Work out the finished part from the listing and answer in its coordinate system (mm). A direction names the side the tool comes from. Round coordinates to 2 decimals unless told otherwise and drop trailing zeros. Order: outer loops, then holes, each group sorted by start corner. A loop starts at its lowest first (then second) coordinate and runs counter-clockwise, first axis right, second up. Notation, with made-up numbers: (68.25, 59.25) - (116.25, 59.25) arc R21 ccw to (116.25, 84.25) - close; hole circle Ø5 at (-18.75, 18). An arc over 180 degrees is marked (long way). Put each result on its own line as item: value.
```python
from build123d import *

# Parameters (mm, degrees)
SKETCH1_W           = 171.075
SKETCH1_H           = 82.339796518
SKETCH1_R           = 10.775
BOSS_EXTRUDE1_DEPTH = 74
SKETCH2_R           = 2.5
CUT_EXTRUDE1_DEPTH  = 12.5


with BuildPart() as part:
    # Sketch1 → Boss-Extrude1 (new body)
    with BuildSketch(Plane(origin=(0, 0, 0), x_dir=(1, 0, 0), z_dir=(0, 1, 0))):
        with Locations((52.9875, 0)):
            Rectangle(SKETCH1_W, SKETCH1_H)
        with Locations(Location((0, 0, 0), (0, 0, 270))):
            Circle(SKETCH1_R, mode=Mode.SUBTRACT)
        with Locations(Location((-11.775, 20.394898259, 0), (0, 0, 270))):
            Circle(SKETCH1_R, mode=Mode.SUBTRACT)
        with Locations(Location((-11.775, -20.394898259, 0), (0, 0, 270))):
            Circle(SKETCH1_R, mode=Mode.SUBTRACT)
        with Locations(Location((11.775, 20.394898259, 0), (0, 0, 270))):
            Circle(SKETCH1_R, mode=Mode.SUBTRACT)
        with Locations(Location((23.55, 0, 0), (0, 0, 270))):
            Circle(SKETCH1_R, mode=Mode.SUBTRACT)
        with Locations(Location((11.775, -20.394898259, 0), (0, 0, 270))):
            Circle(SKETCH1_R, mode=Mode.SUBTRACT)
        with Locations(Location((35.325, 20.394898259, 0), (0, 0, 270))):
            Circle(SKETCH1_R, mode=Mode.SUBTRACT)
        with Locations(Location((47.1, 0, 0), (0, 0, 270))):
            Circle(SKETCH1_R, mode=Mode.SUBTRACT)
        with Locations(Location((35.325, -20.394898259, 0), (0, 0, 270))):
            Circle(SKETCH1_R, mode=Mode.SUBTRACT)
        with Locations(Location((58.875, 20.394898259, 0), (0, 0, 270))):
            Circle(SKETCH1_R, mode=Mode.SUBTRACT)
        with Locations(Location((70.65, 0, 0), (0, 0, 270))):
            Circle(SKETCH1_R, mode=Mode.SUBTRACT)
        with Locations(Location((58.875, -20.394898259, 0), (0, 0, 270))):
            Circle(SKETCH1_R, mode=Mode.SUBTRACT)
        with Locations(Location((82.425, 20.394898259, 0), (0, 0, 270))):
            Circle(SKETCH1_R, mode=Mode.SUBTRACT)
        with Locations(Location((94.2, 0, 0), (0, 0, 270))):
            Circle(SKETCH1_R, mode=Mode.SUBTRACT)
        with Locations(Location((82.425, -20.394898259, 0), (0, 0, 270))):
            Circle(SKETCH1_R, mode=Mode.SUBTRACT)
        with Locations(Location((105.975, 20.394898259, 0), (0, 0, 270))):
            Circle(SKETCH1_R, mode=Mode.SUBTRACT)
        with Locations(Location((117.75, 0, 0), (0, 0, 270))):
            Circle(SKETCH1_R, mode=Mode.SUBTRACT)
        with Locations(Location((105.975, -20.394898259, 0), (0, 0, 270))):
            Circle(SKETCH1_R, mode=Mode.SUBTRACT)
    extrude(amount=BOSS_EXTRUDE1_DEPTH)

    # Sketch2 → Cut-Extrude1 (cut)
    with BuildSketch(Plane.ZY.offset(32.55)):
        with Locations((-37.329831377, 70.010492375)):
            Circle(SKETCH2_R)
        with Locations((36.747951512, 70.905692168)):
            Circle(SKETCH2_R)
        with Locations((34.733751977, 6.451307056)):
            Circle(SKETCH2_R)
        with Locations((-37.777431274, 5.645627242)):
            Circle(SKETCH2_R)
    extrude(amount=-CUT_EXTRUDE1_DEPTH, mode=Mode.SUBTRACT)


solid = part.part
```
1) For faces 5 (the flat face through (-20.05, 70, -37)), 6 (the flat face through (52, 74, -10)), determine the directions among +Z, -Z, +X, -X, +Y, -Y from which every point of the face is accessible in a straight line to the end or side of a thin tool.
Findings below:
face 5: -X
face 6: +Z, -Z, +X, -X, +Y
2) Given pin 1 Ø4.5 at (y, z) = (5.65, -37.78) entering from -X, flat-ended and moving along its own axis, determine where the tip first touches the part or whether it passes through.
Findings below:
pin 1: stops at x = -20.05
3) A cutting plane is placed at A-A on z = 0. Write down the section's boundary in (x, y) (3 decimals), then the cut area to 3 significant figures.
Findings below:
outline: (-32.55, 0) - (-10.775, 0) - (-10.775, 74) - (-32.55, 74) - close; (10.775, 0) - (12.775, 0) - (12.775, 74) - (10.775, 74) - close; (34.325, 0) - (36.325, 0) - (36.325, 74) - (34.325, 74) - close; (57.875, 0) - (59.875, 0) - (59.875, 74) - (57.875, 74) - close; (81.425, 0) - (83.425, 0) - (83.425, 74) - (81.425, 74) - close; (104.975, 0) - (106.975, 0) - (106.975, 74) - (104.975, 74) - close; (128.525, 0) - (138.525, 0) - (138.525, 74) - (128.525, 74) - close
area: 3,090 mm2
4) A cutting plane is placed at C-C on z = 14. Write down the section's boundary in (x, y) (3 decimals), then the cut area to 3 significant figures.
Findings below:
outline: (-32.55, 0) - (-20.447, 0) - (-20.447, 74) - (-32.55, 74) - close; (-3.103, 0) - (3.103, 0) - (3.103, 74) - (-3.103, 74) - close; (20.447, 0) - (26.653, 0) - (26.653, 74) - (20.447, 74) - close; (43.997, 0) - (50.203, 0) - (50.203, 74) - (43.997, 74) - close; (67.547, 0) - (73.753, 0) - (73.753, 74) - (67.547, 74) - close; (91.097, 0) - (97.303, 0) - (97.303, 74) - (91.097, 74) - close; (114.647, 0) - (138.525, 0) - (138.525, 74) - (114.647, 74) - close
area: 4,960 mm2
5) A cutting plane is placed at B-B on x = 43. Write down the section's boundary in (y, z), then the cut area to 3 significant figures.
Findings below:
outline: (0, -41.17) - (74, -41.17) - (74, -27.96) - (0, -27.96) - close; (0, -12.83) - (74, -12.83) - (74, -9.96) - (0, -9.96) - close; (0, 9.96) - (74, 9.96) - (74, 12.83) - (0, 12.83) - close; (0, 27.96) - (74, 27.96) - (74, 41.17) - (0, 41.17) - close
area: 2,380 mm2
6) For a pull along X with two mould halves and no side action, classify faces 1 (the cylindrical face through (-26.387, 4.688, -35.468)), 2 (the flat face through (138.525, 36, 1)), 3 (the cylindrical face through (85.662, 36.482, -10.117)), 4 (the flat face through (-20.05, 71, 37)) as pulls with the +X half, pulls with the -X half, needs draft (parallel to the pull), parting line crosses it, or undercut.
Findings below:
face 1: needs draft
face 2: pulls with the +X half
face 3: undercut
face 4: pulls with the -X half
7) A cutting plane is placed at D-D on y = 23. Give the number of separate pieces and of enclosed holes in the cut face, then the cut area to 3 significant figures.
Findings below:
separate pieces: 1
enclosed holes: 18
area: 7,520 mm2
8) Straight lines are drawn through the part: L1, parallel to Z at x = 71.5, y = 70; L2, parallel to Z at x = 56.5, y = 5; L3, parallel to Z at x = 94.5, y = 70. For each, find the intervals that lie inside material, in ascending order. Write a range as from..to.
Findings below:
L1: z = -41.17..-10.74, 10.74..41.17
L2: z = -41.17..-30.9, -9.88..-5.27, 5.27..9.88, 30.9..41.17
L3: z = -41.17..-10.77, 10.77..41.17
